The listing builds one solid part. Answer for the finished solid, in the listing's coordinates (mm). A direction names the side the tool comes from. Coordinates: 2 decimals unless noted, no trailing zeros. Order: outer loops, then holes, each group sorted by start corner. A loop starts at its lowest first (then second) coordinate and runs counter-clockwise, first axis right, second up. Notation, with made-up numbers: (43, -4.5) - (94, -4.5) arc R15 ccw to (94, 23.5) - close; hole circle Ø7 at (2, 15.25). An arc over 180 degrees is marked (long way). Use a Markdown table: item, result. Add a question column.
Item 1: The mould has two halves that part along Y. Classify faces 1 (the cylindrical face through (4.93, 221.41, -219.82)), 2 (the cylindrical face through (4.93, -34.103, 138.402)): released by +Y, released by -Y, zero draft, split by the parting line, or undercut.
Item 2: The part is cut by section A-A, the plane y = 0. Give the vertices of the cut face in (x, z), then the cut area to 4 significant figures.
Item 3: The part is cut by section B-B, the plane z = -31. Give the vertices of the cut face in (x, y).
Item 4: Flat-ended cylindrical pins translate along their axes: P1, Ø8, axis at y = 20.08, z = -146.13, coming from the -X side; P2, Ø1.5, axis at x = 4, z = -170, coming from the +Y side; P3, Ø5, axis at x = 5.5, y = -191.5, coming from the +Z side. Find the tip coordinate at first contact, or state that the pin passes through.
Item 5: The part is cut by section C-C, the plane x = 4.5. State how many separate pieces and enclosed holes the cut face has, then the cut area to 3 significant figures.
Item 6: Find the intervals of material crossed by line 1 along Z through (x, y) = (4, -66); line 2 along Y through (x, z) = (8.75, 25); line 3 along Z through (x, y) = (1, 169), in increasing order.
Item 7: For faces 3 (the cylindrical face through (4.93, 219.82, 221.41)), 4 (the cylindrical face through (4.93, 209.998, -0.99)), determine the directions among +Z, -Z, +X, -X, +Y, -Y from which every point of the face is accessible in a straight line to the end or side of a thin tool.
from build123d import *

# Parameters (mm, degrees)
ESQUISSE1_R        = 210
ESQUISSE1_R_2      = 6.75
BOSS_EXTRU_1_DEPTH = 10
ESQUISSE2_R        = 41.5
ESQUISSE2_R_2      = 6.75
BOSS_EXTRU_2_DEPTH = 10
BOSS_EXTRU_3_DEPTH = 10
CONG_1_R           = 20


with BuildPart() as part:
    # Esquisse1 → Boss.-Extru.1 (new body)
    with BuildSketch(Plane(origin=(0, 0, 0), x_dir=(0, 0, -1), z_dir=(1, 0, 0))):
        Circle(ESQUISSE1_R)
        with Locations((-147.5, 0)):
            Circle(ESQUISSE1_R_2, mode=Mode.SUBTRACT)
        with Locations((-142.030299884, 39.795023746)):
            Circle(ESQUISSE1_R_2, mode=Mode.SUBTRACT)
        with Locations((-126.026862171, 76.63863263)):
            Circle(ESQUISSE1_R_2, mode=Mode.SUBTRACT)
        with Locations((-100.676588625, 107.798304731)):
            Circle(ESQUISSE1_R_2, mode=Mode.SUBTRACT)
        with Locations((-67.859593065, 130.963069714)):
            Circle(ESQUISSE1_R_2, mode=Mode.SUBTRACT)
        with Locations((49.394742795, 138.983486013)):
            Circle(ESQUISSE1_R_2, mode=Mode.SUBTRACT)
        with Locations((85.060347512, 120.503059219)):
            Circle(ESQUISSE1_R_2, mode=Mode.SUBTRACT)
        with Locations((114.417415379, 93.085471788)):
            Circle(ESQUISSE1_R_2, mode=Mode.SUBTRACT)
        with Locations((135.288666972, 58.764160752)):
            Circle(ESQUISSE1_R_2, mode=Mode.SUBTRACT)
        with Locations((146.12617704, 20.084580742)):
            Circle(ESQUISSE1_R_2, mode=Mode.SUBTRACT)
        with Locations((146.12617704, -20.084580742)):
            Circle(ESQUISSE1_R_2, mode=Mode.SUBTRACT)
        with Locations((135.288666972, -58.764160752)):
            Circle(ESQUISSE1_R_2, mode=Mode.SUBTRACT)
        with Locations((114.417415379, -93.085471788)):
            Circle(ESQUISSE1_R_2, mode=Mode.SUBTRACT)
        with Locations((85.060347512, -120.503059219)):
            Circle(ESQUISSE1_R_2, mode=Mode.SUBTRACT)
        with Locations((49.394742795, -138.983486013)):
            Circle(ESQUISSE1_R_2, mode=Mode.SUBTRACT)
        with Locations((-67.859593065, -130.963069714)):
            Circle(ESQUISSE1_R_2, mode=Mode.SUBTRACT)
        with Locations((-100.676588625, -107.798304731)):
            Circle(ESQUISSE1_R_2, mode=Mode.SUBTRACT)
        with Locations((-126.026862171, -76.63863263)):
            Circle(ESQUISSE1_R_2, mode=Mode.SUBTRACT)
        with Locations((-142.030299884, -39.795023746)):
            Circle(ESQUISSE1_R_2, mode=Mode.SUBTRACT)
        with BuildLine():
            Line((40, -130), (40, -126.318050967))
            ThreePointArc((40, -126.318050967), (132.5, 0), (40, 126.318050967))
            Line((40, 126.318050967), (40, 130))
            Line((40, 130), (40, 170))
            Line((40, 170), (-40, 170))
            Line((-40, 170), (-40, 130))
            Line((-40, 130), (-40, 126.318050967))
            ThreePointArc((-40, 126.318050967), (-132.5, 0), (-40, -126.318050967))
            Line((-40, -126.318050967), (-40, -130))
            Line((-40, -130), (-40, -170))
            Line((-40, -170), (40, -170))
            Line((40, -170), (40, -130))
        make_face(mode=Mode.SUBTRACT)
    extrude(amount=BOSS_EXTRU_1_DEPTH)

    # Esquisse2 → Boss.-Extru.2 (add)
    # profile 1 of 4: a face of its own
    with BuildSketch(Plane.ZY):
        with BuildLine():
            Line((-156.896697906, -269.680229505), (-80.976239027, -193.759770626))
            ThreePointArc((-80.976239027, -193.759770626), (-148.492424049, -148.492424049), (-193.759770626, -80.976239027))
            Line((-193.759770626, -80.976239027), (-269.680229505, -156.896697906))
            ThreePointArc((-269.680229505, -156.896697906), (-220.61731573, -220.61731573), (-156.896697906, -269.680229505))
        make_face()
        with Locations((-180.665782593, -180.665782593)):
            Circle(ESQUISSE2_R, mode=Mode.SUBTRACT)
        with Locations((-143.18912319, -218.142441996)):
            Circle(ESQUISSE2_R_2, mode=Mode.SUBTRACT)
        with Locations((-218.142441996, -143.18912319)):
            Circle(ESQUISSE2_R_2, mode=Mode.SUBTRACT)
    # profile 2 of 4: a face of its own
    with BuildSketch(Plane.ZY):
        with BuildLine():
            Line((80.976239027, -193.759770626), (156.896697906, -269.680229505))
            ThreePointArc((156.896697906, -269.680229505), (220.61731573, -220.61731573), (269.680229505, -156.896697906))
            Line((269.680229505, -156.896697906), (193.759770626, -80.976239027))
            ThreePointArc((193.759770626, -80.976239027), (148.492424049, -148.492424049), (80.976239027, -193.759770626))
        make_face()
        with Locations((143.18912319, -218.142441996)):
            Circle(ESQUISSE2_R_2, mode=Mode.SUBTRACT)
        with Locations((180.665782593, -180.665782593)):
            Circle(ESQUISSE2_R, mode=Mode.SUBTRACT)
        with Locations((218.142441996, -143.18912319)):
            Circle(ESQUISSE2_R_2, mode=Mode.SUBTRACT)
    # profile 3 of 4: a face of its own
    with BuildSketch(Plane.ZY):
        with BuildLine():
            Line((-269.680229505, 156.896697906), (-193.759770626, 80.976239027))
            ThreePointArc((-193.759770626, 80.976239027), (-148.492424049, 148.492424049), (-80.976239027, 193.759770626))
            Line((-80.976239027, 193.759770626), (-156.896697906, 269.680229505))
            ThreePointArc((-156.896697906, 269.680229505), (-220.61731573, 220.61731573), (-269.680229505, 156.896697906))
        make_face()
        with Locations((-218.142441996, 143.18912319)):
            Circle(ESQUISSE2_R_2, mode=Mode.SUBTRACT)
        with Locations((-180.665782593, 180.665782593)):
            Circle(ESQUISSE2_R, mode=Mode.SUBTRACT)
        with Locations((-143.18912319, 218.142441996)):
            Circle(ESQUISSE2_R_2, mode=Mode.SUBTRACT)
    # profile 4 of 4: a face of its own
    with BuildSketch(Plane.ZY):
        with BuildLine():
            ThreePointArc((269.680229505, 156.896697906), (220.61731573, 220.61731573), (156.896697906, 269.680229505))
            Line((156.896697906, 269.680229505), (80.976239027, 193.759770626))
            ThreePointArc((80.976239027, 193.759770626), (148.492424049, 148.492424049), (193.759770626, 80.976239027))
            Line((193.759770626, 80.976239027), (269.680229505, 156.896697906))
        make_face()
        with Locations((218.142441996, 143.18912319)):
            Circle(ESQUISSE2_R_2, mode=Mode.SUBTRACT)
        with Locations((143.18912319, 218.142441996)):
            Circle(ESQUISSE2_R_2, mode=Mode.SUBTRACT)
        with Locations((180.665782593, 180.665782593)):
            Circle(ESQUISSE2_R, mode=Mode.SUBTRACT)
    extrude(amount=-BOSS_EXTRU_2_DEPTH)

    # Esquisse3 → Boss.-Extru.3 (add)
    with BuildSketch(Plane(origin=(10, 0, 0), x_dir=(0, 0, -1), z_dir=(1, 0, 0))):
        Polygon((-156.896697906, -269.680229505), (156.896697906, -269.680229505), (126.896697906, -239.680229505), (-126.896697906, -239.680229505), align=None)
        Polygon((-269.680229505, -156.896697906), (-269.680229505, 156.896697906), (-239.680229505, 126.896697906), (-239.680229505, -126.896697906), align=None)
        Polygon((-156.896697906, 269.680229505), (156.896697906, 269.680229505), (126.896697906, 239.680229505), (-126.896697906, 239.680229505), align=None)
        Polygon((269.680229505, 156.896697906), (269.680229505, -156.896697906), (239.680229505, -126.896697906), (239.680229505, 126.896697906), align=None)
    extrude(amount=-BOSS_EXTRU_3_DEPTH)

    # Congé1
    cong_1_edges = [part.edges().sort_by_distance(p)[0] for p in [
        (5, -193.759770626, 80.976239027),
        (5, -80.976239027, 193.759770626),
        (5, 80.976239027, 193.759770626),
        (5, 193.759770626, 80.976239027),
        (5, 193.759770626, -80.976239027),
        (5, 80.976239027, -193.759770626),
        (5, -80.976239027, -193.759770626),
        (5, -193.759770626, -80.976239027),
        (5, -239.680229505, 126.896697906),
        (5, -239.680229505, -126.896697906),
        (5, -126.896697906, 239.680229505),
        (5, 126.896697906, 239.680229505),
        (5, 239.680229505, 126.896697906),
        (5, 239.680229505, -126.896697906),
        (5, 126.896697906, -239.680229505),
        (5, -126.896697906, -239.680229505),
    ]]
    fillet(cong_1_edges, radius=CONG_1_R)


solid = part.part
Solution:
| question | item | result |
|---|---|---|
| 1 | face 1 | released by +Y |
| 1 | face 2 | undercut |
| 2 | outline | (0, -269.68) - (10, -269.68) - (10, -239.68) - (0, -239.68) - close; (0, -210) - (10, -210) - (10, -132.5) - (0, -132.5) - close; (0, 132.5) - (10, 132.5) - (10, 140.75) - (0, 140.75) - close; (0, 154.25) - (10, 154.25) - (10, 210) - (0, 210) - close; (0, 239.68) - (10, 239.68) - (10, 269.68) - (0, 269.68) - close |
| 2 | area | 2,015 mm2 |
| 3 | outline | (0, -269.68) - (10, -269.68) - (10, -239.68) - (0, -239.68) - close; (0, -207.7) - (10, -207.7) - (10, -170) - (0, -170) - close; (0, 170) - (10, 170) - (10, 207.7) - (0, 207.7) - close; (0, 239.68) - (10, 239.68) - (10, 269.68) - (0, 269.68) - close |
| 4 | P1 | passes through |
| 4 | P2 | stops at y = 262.1 |
| 4 | P3 | stops at z = 248.24 |
| 5 | separate pieces | 1 |
| 5 | enclosed holes | 36 |
| 5 | area | 156,000 mm2 |
| 6 | line 1 | z = -269.68 to -239.68, -199.36 to -114.89, 114.89 to 199.36, 239.68 to 269.68 |
| 6 | line 2 | y = -269.68 to -239.68, -208.51 to -170, 170 to 208.51, 239.68 to 269.68 |
| 6 | line 3 | z = -262.27 to -220.49, -140.84 to -40, 40 to 140.84, 220.49 to 262.27 |
| 7 | face 3 | +Z, +X, -X, +Y |
| 7 | face 4 | +X, -X |
